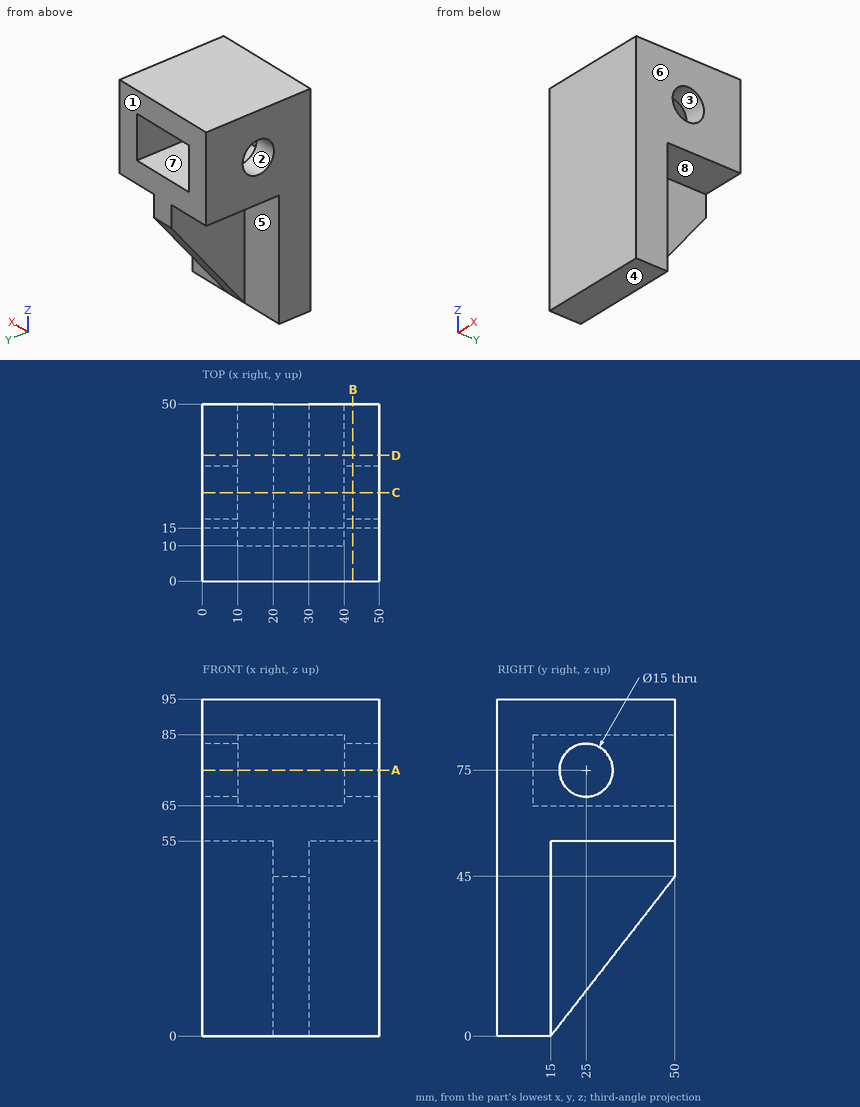
Job drawing, mm, ordinate dimensions from the low corner. One solid piece. A direction names the side the tool comes from. Give positions to 0.01 mm unless a question says otherwise; leave off trailing zeros. Write each loop counter-clockwise with the first axis right and the second up, starting at its lowest first coordinate (ties: lowest second). Pieces come first, ordered by that corner, then holes. Notation, with made-up numbers: (27, 77) -> (77, 77) arc R10 cw to (77, 93) -> close; hole circle Ø7 at (-15, 13). An arc over 180 degrees is marked (long way). Return JSON: item names as keys, results as strings.
Item 1: Drop flat-ended pins along their axis: pin 1 (16 mm diameter, centred on x = 39, y = 28, fed in from -Z); pin 2 (1 mm diameter, centred on x = 14.5, z = 51, fed in from +Y); pin 3 (17.5 mm diameter, centred on y = 39.5, z = 37.5, fed in from -X). Give the stop position or say it passes through.
Answer below:
{"pin 1": "stops at z = 55", "pin 2": "stops at y = 15", "pin 3": "stops at x = 20"}
Item 2: Tool access for the marked faces 5, 6, 7 and 8: list every direction of +Z, -Z, +X, -X, +Y, -Y with a clear straight run to the whole face (end or side of a thin tool).
Answer below:
{"face 5": "-Z, -X, +Y", "face 6": "+Z, -Z, +X, +Y, -Y", "face 7": "+Y", "face 8": "-Z, +X, +Y"}
Item 3: Two-plate mould, pull along Y, no slides. Class the marked faces 1, 2, 3 and 4: +Y half, -Y half, draft (parallel to the pull), parting line (faces both ways), or undercut.
Answer below:
{"face 1": "+Y half", "face 2": "undercut", "face 3": "undercut", "face 4": "draft"}
Item 4: Band-saw the part on B-B (x = 42.5). List the corners of the cut face in (y, z), then the cut area to 3 significant figures.
Answer below:
{"outline": "(0, 0) -> (15, 0) -> (15, 55) -> (50, 55) -> (50, 95) -> (0, 95) -> close; hole circle Ø15 at (25, 75)", "area": "2,650 mm2"}
Item 5: Band-saw the part on C-C (y = 25). List the corners of the cut face in (x, z).
Answer below:
{"outline": "(0, 55) -> (20, 55) -> (20, 12.86) -> (30, 12.86) -> (30, 55) -> (50, 55) -> (50, 67.5) -> (40, 67.5) -> (40, 65) -> (10, 65) -> (10, 67.5) -> (0, 67.5) -> close; (0, 82.5) -> (10, 82.5) -> (10, 85) -> (40, 85) -> (40, 82.5) -> (50, 82.5) -> (50, 95) -> (0, 95) -> close"}
Item 6: Drill centre lines: probe 1 along Y at (x, z) = (4.5, 75); probe 2 along Z at (x, y) = (8, 25); probe 3 along X at (y, z) = (13, 71.5). Where is each one in solid material? Low to high.
Answer below:
{"probe 1": "y = 0 to 17.5, 32.5 to 50", "probe 2": "z = 55 to 67.5, 82.5 to 95", "probe 3": "x = 0 to 10, 40 to 50"}
Item 7: Band-saw the part on A-A (z = 75). List the corners of the cut face in (x, y).
Answer below:
{"outline": "(0, 0) -> (50, 0) -> (50, 17.5) -> (40, 17.5) -> (40, 10) -> (10, 10) -> (10, 17.5) -> (0, 17.5) -> close; (0, 32.5) -> (10, 32.5) -> (10, 50) -> (0, 50) -> close; (40, 32.5) -> (50, 32.5) -> (50, 50) -> (40, 50) -> close"}
Item 8: Band-saw the part on D-D (y = 35.5). List the corners of the cut face in (x, z).
Answer below:
{"outline": "(0, 55) -> (20, 55) -> (20, 26.36) -> (30, 26.36) -> (30, 55) -> (50, 55) -> (50, 95) -> (0, 95) -> close; hole (10, 65) -> (40, 65) -> (40, 85) -> (10, 85) -> close"}
